Here's how the part is built. I have some questions about the finished solid (model axes, mm). Round coordinates to 2 decimals unless told otherwise and drop trailing zeros. Write each loop counter-clockwise with the first axis right and the second up, starting at its lowest first coordinate (ties: lowest second). Pieces come first, ordered by that corner, then holes. Notation, with made-up numbers: (-14.75, 45) - (18.25, 45) arc R26 ccw to (18.25, 83) - close; hole circle Ø10 at (82.5, -15.5). An arc over 180 degrees is marked (long way). Write item = value, one per line. Start each with the question number.
Item 1: For P1, Ø2, axis at y = 0, z = -1, coming from the -X side, with a flat end and sliding along its axis, tell me the tip position at first contact or that it passes through.
Item 2: If I drill on line 1 along Z through (x, y) = (0, -1.5); line 2 along Y through (x, z) = (-1.65, -0.6); line 3 along Z through (x, y) = (0.55, 1.25), over which ranges is the centre line in solid material (lowest first)? Write a range as [from, to].
Item 3: If we section it at A-A (y = -0.5): Please give me the cut outline in (x, z), and give its area (3 significant figures).
```python
from build123d import *
from build123d.topology import SkipClean

# Parameters (mm, degrees)
SKETCH1_R           = 1.5
BOSS_EXTRUDE1_DEPTH = 2
SKETCH2_R           = 2
BOSS_EXTRUDE2_DEPTH = 1.5
FILLET1_R           = 1
FILLET2_R           = 0.2


# Read off the part's stored shape, not the designer's step: Mirror2
with BuildPart() as part:
    # Sketch1 → Boss-Extrude1 (new body)
    with BuildSketch(Plane(origin=(0, 0, 0), x_dir=(1, 0, 0), z_dir=(0, 1, 0))):
        with Locations(Location((0, 0, 0), (0, 0, 270))):
            Circle(SKETCH1_R)
    extrude(amount=BOSS_EXTRUDE1_DEPTH)

    # Sketch2 → Boss-Extrude2 (add)
    with BuildSketch(Plane(origin=(0, 2, 0), x_dir=(1, 0, 0), z_dir=(0, 1, 0))):
        with Locations(Location((0, 0, 0), (0, 0, 270))):
            Circle(SKETCH2_R)
    extrude(amount=BOSS_EXTRUDE2_DEPTH)

    # Fillet1
    fillet1_edges = [part.edges().sort_by_distance(p)[0] for p in [
        (0, 3.5, -2),
    ]]
    fillet(fillet1_edges, radius=FILLET1_R)

    # Fillet2
    fillet2_edges = [part.edges().sort_by_distance(p)[0] for p in [
        (0, 2, -2),
    ]]
    fillet(fillet2_edges, radius=FILLET2_R)

    # Mirror2 outline → Mirror2 (revolve)
    with SkipClean():  # the faces are left unmerged after this step: merging them gives an invalid solid
        with BuildSketch(Plane.XY):
            with BuildLine():
                Line((1.5, -2), (1.5, 0))
                Line((1.5, 0), (0, 0))
                Line((0, 0), (0, -3.5))
                Line((0, -3.5), (1, -3.5))
                ThreePointArc((1, -3.5), (1.707106781, -3.207106781), (2, -2.5))
                Line((2, -2.5), (2, -2.2))
                ThreePointArc((2, -2.2), (1.941421356, -2.058578644), (1.8, -2))
                Line((1.8, -2), (1.5, -2))
            make_face()
        revolve(axis=Axis((0, 0, 0), (0, 1, 0)))
    add(part.part.scale(1), mode=Mode.REPLACE)  # the faces are merged on a copy


solid = part.part
```
Reply:
q1.P1 = -1.5
q2.line_1 = [-1.5, 1.5]
q2.line_2 = [-3.15, -2], [2, 3.15]
q2.line_3 = [-1.4, 1.4]
q3.outline = circle Ø3 at (0, 0)
q3.area = 7.07 mm2
